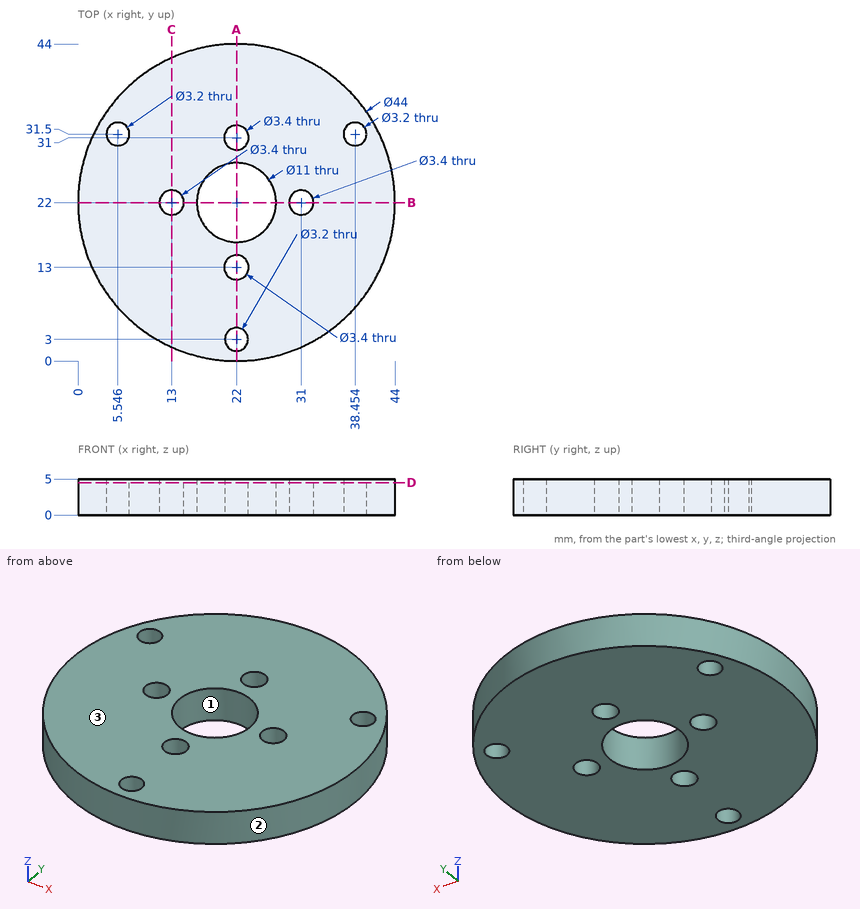
Job drawing, mm, ordinate dimensions from the low corner. One solid piece. Coordinates: 2 decimals unless noted, no trailing zeros. Loops run counter-clockwise (first coordinate to the right, second up) from the corner with the lowest first, then second, coordinate; pieces in that order, holes last. Notation, with made-up numbers: (71, 5) - (90, 5) arc R10 ccw to (90, 11) - close; hole circle Ø6 at (62, 81.25). An arc over 180 degrees is marked (long way). Answer as a JSON object with one key per item and string values. Group by question number.
(1) Cut at D-D (z = 4.5). State how many separate pieces and enclosed holes the cut face has, then the cut area to 4 significant figures.
(2) Cut at A-A (x = 22). Give the cut face in (y, z).
(3) Probe line 1 along Y through (x, z) = (22, 2.85); line 2 along Y through (x, z) = (32, 3.55) (1 decimal); line 3 along Y through (x, z) = (13, 3.85) (1 decimal). List the from-to ranges inside material, lowest first.
(4) Two-plate mould, pull along Y, no slides. Class the marked faces 1, 2 and 3: released by +Y, released by -Y, zero draft, split by the parting line, or undercut.
(5) Cut at B-B (y = 22). Give the cut face in (x, z).
(6) Cut at C-C (x = 13). Give the cut face in (y, z) (1 decimal), then the cut area to 3 significant figures.
(7) Flat gauge pins, fed straight in: pin 1 (3 mm diameter, centred on y = 19, z = 3, fed in from -X); pin 2 (1 mm diameter, centred on y = 12.5, z = 1, fed in from +X) (1 decimal); pin 3 (3 mm diameter, centred on x = 4.5, z = 1, fed in from +Y); pin 4 (5 mm diameter, centred on x = 5.55, y = 31.5, fed in from +Z). Where does each tip first touch, or does it go through?
Geometry says:
{
 "1": {"separate pieces": "1", "enclosed holes": "8", "area": "1,365 mm^2"},
 "2": {"outline": "(0, 0) - (1.4, 0) - (1.4, 5) - (0, 5) - close; (4.6, 0) - (11.3, 0) - (11.3, 5) - (4.6, 5) - close; (14.7, 0) - (16.5, 0) - (16.5, 5) - (14.7, 5) - close; (27.5, 0) - (29.3, 0) - (29.3, 5) - (27.5, 5) - close; (32.7, 0) - (44, 0) - (44, 5) - (32.7, 5) - close"},
 "3": {"line 1": "y = 0 to 1.4, 4.6 to 11.3, 14.7 to 16.5, 27.5 to 29.3, 32.7 to 44", "line 2": "y = 2.4 to 20.6, 23.4 to 41.6", "line 3": "y = 1.9 to 20.3, 23.7 to 42.1"},
 "4": {"face 1": "undercut", "face 2": "split by the parting line", "face 3": "zero draft"},
 "5": {"outline": "(0, 0) - (11.3, 0) - (11.3, 5) - (0, 5) - close; (14.7, 0) - (16.5, 0) - (16.5, 5) - (14.7, 5) - close; (27.5, 0) - (29.3, 0) - (29.3, 5) - (27.5, 5) - close; (32.7, 0) - (44, 0) - (44, 5) - (32.7, 5) - close"},
 "6": {"outline": "(1.9, 0) - (20.3, 0) - (20.3, 5) - (1.9, 5) - close; (23.7, 0) - (42.1, 0) - (42.1, 5) - (23.7, 5) - close", "area": "184 mm^2"},
 "7": {"pin 1": "stops at x = 0.05", "pin 2": "stops at x = 42.1", "pin 3": "stops at y = 37.1", "pin 4": "stops at z = 5"}
}
